```python
from build123d import *

# Parameters (mm, degrees)
SKETCH3_R           = 8.99999978
SKETCH3_R_2         = 1.49999954
BOSS_EXTRUDE1_DEPTH = 2


with BuildPart() as part:
    # Sketch3 → Boss-Extrude1 (new body)
    with BuildSketch(Plane.XY):
        with BuildLine():
            Line((75.5000014, 79.49999848), (75.5000014, 94.49999896))
            ThreePointArc((75.5000014, 94.49999896), (90.50000188, 109.49999944), (105.50000236, 94.49999896))
            Line((105.50000236, 94.49999896), (105.50000236, 66.99999808))
            ThreePointArc((105.50000236, 66.99999808), (104.76776929, 65.23223107), (103.00000228, 64.499998))
            Line((103.00000228, 64.499998), (78.00000148, 64.499998))
            ThreePointArc((78.00000148, 64.499998), (76.23223447, 65.23223107), (75.5000014, 66.99999808))
            Line((75.5000014, 66.99999808), (75.5000014, 79.49999848))
        make_face()
        with Locations((90.50000188, 94.49999896)):
            Circle(SKETCH3_R, mode=Mode.SUBTRACT)
        with Locations((90.50000188, 69.49999816)):
            Circle(SKETCH3_R_2, mode=Mode.SUBTRACT)
    extrude(amount=BOSS_EXTRUDE1_DEPTH)


solid = part.part
```
The listing builds one solid part. Answer for the finished solid, in the listing's coordinates (mm). Round coordinates to 2 decimals unless told otherwise and drop trailing zeros. Order: outer loops, then holes, each group sorted by start corner. A loop starts at its lowest first (then second) coordinate and runs counter-clockwise, first axis right, second up. Notation, with made-up numbers: (6, 45.5) - (38, 45.5) arc R20 ccw to (38, 52.5) - close; hole circle Ø2 at (-35, 68). An arc over 180 degrees is marked (long way). Put each result on its own line as item: value. Start each with the question number.
(1) Given P1, Ø10, axis at x = 80, y = 71.5, coming from the -Z side, flat-ended and moving along its own axis, determine where the tip first touches the part or whether it passes through.
(2) Determine the mould class of faces 1 (the cylindrical face through (90.17, 109.496, 0.986)), 2 (the flat face through (91, 82, 2)), 3 (the cylindrical face through (83.867, 100.583, 0.986)), 4 (the cylindrical face through (76.252, 65.213, 0.986)) for opening direction Y: released by +Y, released by -Y, zero draft, split by the parting line, or undercut.
(3) Find section B-B (y = 70). Give the vertices of the cut face in (x, z).
(4) Find section A-A (z = 0.85). Give the vertices of the cut face in (x, y).
(5) Find section D-D (x = 85.5). Give the vertices of the cut face in (y, z), plus the area to 3 significant figures.
(6) Straight lines are drawn through the part: probe 1 along Y at (x, z) = (91, 0.2); probe 2 along Y at (x, z) = (89.5, 1.15); probe 3 along Y at (x, z) = (78.5, 1.5). For each, find the intervals that lie inside material, in ascending order. Write a range as from..to.
(7) Find section C-C (x = 91). Give the vertices of the cut face in (y, z), plus the area to 3 significant figures.
Reply:
1. P1: z = 0
2. face 1: released by +Y
2. face 2: zero draft
2. face 3: undercut
2. face 4: released by -Y
3. outline: (75.5, 0) - (89.09, 0) - (89.09, 2) - (75.5, 2) - close; (91.91, 0) - (105.5, 0) - (105.5, 2) - (91.91, 2) - close
4. outline: (75.5, 67) arc R2.5 ccw to (78, 64.5) - (103, 64.5) arc R2.5 ccw to (105.5, 67) - (105.5, 94.5) arc R15 ccw to (75.5, 94.5) - close; hole circle Ø18 at (90.5, 94.5); hole circle Ø3 at (90.5, 69.5)
5. outline: (64.5, 0) - (87.02, 0) - (87.02, 2) - (64.5, 2) - close; (101.98, 0) - (108.64, 0) - (108.64, 2) - (101.98, 2) - close
5. area: 58.4 mm^2
6. probe 1: 64.5..68.09, 70.91..85.51, 103.49..109.49
6. probe 2: 64.5..68.38, 70.62..85.56, 103.44..109.47
6. probe 3: 64.5..103.5
7. outline: (64.5, 0) - (68.09, 0) - (68.09, 2) - (64.5, 2) - close; (70.91, 0) - (85.51, 0) - (85.51, 2) - (70.91, 2) - close; (103.49, 0) - (109.49, 0) - (109.49, 2) - (103.49, 2) - close
7. area: 48.4 mm^2
